Design review of the part built by this model. Coordinates are the model's own, in mm. Give positions to 0.01 mm unless a question says otherwise; leave off trailing zeros. Write each loop counter-clockwise with the first axis right and the second up, starting at its lowest first coordinate (ties: lowest second). Pieces come first, ordered by that corner, then holes. Notation, with made-up numbers: (-25.75, -27) -> (-8.75, -27) arc R32 cw to (-8.75, 10) -> close; hole circle Ø2 at (-17.75, 45). An arc over 180 degrees is marked (long way). Answer as a JSON object with one key per item and string values.
```python
from build123d import *

# Parameters (mm, degrees)
BOSS_EXTRUDE1_DEPTH     = 5
BOSS_EXTRUDE2_START     = 250
BOSS_EXTRUDE2_DEPTH     = 5
BOSS_EXTRUDE3_DEPTH     = 5
BOSS_EXTRUDE4_DEPTH     = 5
BOSS_EXTRUDE5_START     = -2.5
SKETCH12_R              = 5
BOSS_EXTRUDE5_DEPTH     = 2.5
BOSS_EXTRUDE6_START     = -20
SKETCH12_2_R            = 5
BOSS_EXTRUDE6_DEPTH     = 2.5
MIRROR2_START           = 250
MIRROR2_COPY_1_DEPTH    = 5
MIRROR2_COPY_2_DEPTH    = 5
MIRROR2_COPY_3_DEPTH    = 5
MIRROR2_START_2         = -2.5
MIRROR2_COPY_4_SKETCH_R = 5
MIRROR2_COPY_4_DEPTH    = 2.5
MIRROR2_START_3         = -20
MIRROR2_COPY_5_SKETCH_R = 5
MIRROR2_COPY_5_DEPTH    = 2.5
SKETCH13_W              = 25
SKETCH13_H              = 10
CUT_EXTRUDE1_DEPTH      = 5
FILLET1_R               = 2.5
SKETCH15_W              = 25
SKETCH15_H              = 10
CUT_EXTRUDE2_DEPTH      = 5
FILLET2_R               = 2.5


with BuildPart() as part:
    # Sketch2 → Boss-Extrude1 (new body, symmetric)
    with BuildSketch(Plane(origin=(0, 0, 0), x_dir=(1, 0, 0), z_dir=(0, 1, 0))):
        with BuildLine():
            Line((-272.5, 125), (-187.5, 125))
            ThreePointArc((-187.5, 125), (-62.5, 0), (-187.5, -125))
            Line((-187.5, -125), (-272.5, -125))
            ThreePointArc((-272.5, -125), (-300.784271247, -136.715728753), (-312.5, -165))
            Line((-312.5, -165), (-312.5, -175))
            Line((-312.5, -175), (312.5, -175))
            Line((312.5, -175), (312.5, -165))
            ThreePointArc((312.5, -165), (300.784271247, -136.715728753), (272.5, -125))
            Line((272.5, -125), (187.5, -125))
            ThreePointArc((187.5, -125), (62.5, 0), (187.5, 125))
            Line((187.5, 125), (272.5, 125))
            ThreePointArc((272.5, 125), (300.784271247, 136.715728753), (312.5, 165))
            Line((312.5, 165), (312.5, 175))
            Line((312.5, 175), (-312.5, 175))
            Line((-312.5, 175), (-312.5, 165))
            ThreePointArc((-312.5, 165), (-300.784271247, 136.715728753), (-272.5, 125))
        make_face()
    extrude(amount=BOSS_EXTRUDE1_DEPTH, both=True)

    # Sketch5 → Boss-Extrude2 (add)
    with BuildSketch(Plane(origin=(0, 0, 0), x_dir=(0, 0, -1), z_dir=(1, 0, 0)).offset(BOSS_EXTRUDE2_START)):
        with BuildLine():
            Line((175, 5), (125, 5))
            ThreePointArc((125, 5), (143.63387523, 48.296145769), (150, 95))
            Line((150, 95), (175, 95))
            Line((175, 95), (175, 5))
        make_face()
    boss_extrude2 = extrude(amount=BOSS_EXTRUDE2_DEPTH)

    # Sketch7 → Boss-Extrude3 (add)
    with BuildSketch(Plane(origin=(0, 95, 0), x_dir=(1, 0, 0), z_dir=(0, 1, 0))):
        with BuildLine():
            Line((260, 147.5), (137.5, 147.5))
            ThreePointArc((137.5, 147.5), (135.732233047, 148.232233047), (135, 150))
            Line((135, 150), (135, 155.899029492))
            ThreePointArc((135, 155.899029492), (135.394692651, 157.247243483), (136.454144772, 158.16975335))
            Line((136.454144772, 158.16975335), (172.44973726, 174.748686302))
            ThreePointArc((172.44973726, 174.748686302), (178.575849825, 176.804100302), (185, 177.5))
            Line((185, 177.5), (260, 177.5))
            Line((260, 177.5), (260, 147.5))
        make_face()
    boss_extrude3 = extrude(amount=-BOSS_EXTRUDE3_DEPTH)

    # Sketch10 → Boss-Extrude4 (add)
    with BuildSketch(Plane.ZY.offset(-150)):
        with BuildLine():
            Line((-175, 5), (-125, 5))
            ThreePointArc((-125, 5), (-141.779773176, 46.036236512), (-147.5, 90))
            Line((-147.5, 90), (-164.408734572, 90))
            ThreePointArc((-164.408734572, 90), (-167.06674937, 47.171344571), (-175, 5))
        make_face()
    boss_extrude4 = extrude(amount=-BOSS_EXTRUDE4_DEPTH)

    # Sketch12 → Boss-Extrude5 (add)
    with BuildSketch(Plane.XY.offset(-147.5).offset(BOSS_EXTRUDE5_START)):
        with BuildLine():
            Line((175, 95), (200, 95))
            Line((200, 95), (197.12585943, 105.209765716))
            ThreePointArc((197.12585943, 105.209765716), (187.5, 112.5), (177.87414057, 105.209765716))
            Line((177.87414057, 105.209765716), (175, 95))
        make_face()
        with Locations((187.5, 102.5)):
            Circle(SKETCH12_R, mode=Mode.SUBTRACT)
    boss_extrude5 = extrude(amount=-BOSS_EXTRUDE5_DEPTH)

    # Sketch12<2> → Boss-Extrude6 (add)
    with BuildSketch(Plane.XY.offset(-147.5).offset(BOSS_EXTRUDE6_START)):
        with BuildLine():
            Line((175, 95), (200, 95))
            Line((200, 95), (197.12585943, 105.209765716))
            ThreePointArc((197.12585943, 105.209765716), (187.5, 112.5), (177.87414057, 105.209765716))
            Line((177.87414057, 105.209765716), (175, 95))
        make_face()
        with Locations((187.5, 102.5)):
            Circle(SKETCH12_2_R, mode=Mode.SUBTRACT)
    boss_extrude6 = extrude(amount=-BOSS_EXTRUDE6_DEPTH)

    # Mirror1: Boss-Extrude2, Boss-Extrude3, Boss-Extrude4, Boss-Extrude5, Boss-Extrude6 across plane
    add(boss_extrude2.mirror(Plane.XY))
    add(boss_extrude3.mirror(Plane.XY))
    add(boss_extrude4.mirror(Plane.XY))
    add(boss_extrude5.mirror(Plane.XY))
    add(boss_extrude6.mirror(Plane.XY))

    # Mirror2: Boss-Extrude2, Boss-Extrude3, Boss-Extrude4, Boss-Extrude5, Boss-Extrude6 across plane
    add(boss_extrude2.mirror(Plane(origin=(0, 0, 0), x_dir=(0, 0, 1), z_dir=(1, 0, 0))))
    add(boss_extrude3.mirror(Plane(origin=(0, 0, 0), x_dir=(0, 0, 1), z_dir=(1, 0, 0))))
    add(boss_extrude4.mirror(Plane(origin=(0, 0, 0), x_dir=(0, 0, 1), z_dir=(1, 0, 0))))
    add(boss_extrude5.mirror(Plane(origin=(0, 0, 0), x_dir=(0, 0, 1), z_dir=(1, 0, 0))))
    add(boss_extrude6.mirror(Plane(origin=(0, 0, 0), x_dir=(0, 0, 1), z_dir=(1, 0, 0))))

    # Mirror2 copy 1 sketch → Mirror2 copy 1 (add)
    with BuildSketch(Plane.ZY.offset(MIRROR2_START)):
        with BuildLine():
            Line((175, 5), (125, 5))
            ThreePointArc((125, 5), (143.63387523, 48.296145769), (150, 95))
            Line((150, 95), (175, 95))
            Line((175, 95), (175, 5))
        make_face()
    extrude(amount=MIRROR2_COPY_1_DEPTH)

    # Mirror2 copy 2 sketch → Mirror2 copy 2 (add)
    with BuildSketch(Plane(origin=(0, 95, 0), x_dir=(-1, 0, 0), z_dir=(0, 1, 0))):
        with BuildLine():
            Line((260, 147.5), (137.5, 147.5))
            ThreePointArc((137.5, 147.5), (135.732233047, 148.232233047), (135, 150))
            Line((135, 150), (135, 155.899029492))
            ThreePointArc((135, 155.899029492), (135.394692651, 157.247243483), (136.454144772, 158.16975335))
            Line((136.454144772, 158.16975335), (172.44973726, 174.748686302))
            ThreePointArc((172.44973726, 174.748686302), (178.575849825, 176.804100302), (185, 177.5))
            Line((185, 177.5), (260, 177.5))
            Line((260, 177.5), (260, 147.5))
        make_face()
    extrude(amount=-MIRROR2_COPY_2_DEPTH)

    # Mirror2 copy 3 sketch → Mirror2 copy 3 (add)
    with BuildSketch(Plane(origin=(-150, 0, 0), x_dir=(0, 0, -1), z_dir=(1, 0, 0))):
        with BuildLine():
            Line((-175, 5), (-125, 5))
            ThreePointArc((-125, 5), (-141.779773176, 46.036236512), (-147.5, 90))
            Line((-147.5, 90), (-164.408734572, 90))
            ThreePointArc((-164.408734572, 90), (-167.06674937, 47.171344571), (-175, 5))
        make_face()
    extrude(amount=-MIRROR2_COPY_3_DEPTH)

    # Mirror2 copy 4 sketch → Mirror2 copy 4 (add)
    with BuildSketch(Plane(origin=(0, 0, 147.5), x_dir=(-1, 0, 0), z_dir=(0, 0, -1)).offset(MIRROR2_START_2)):
        with BuildLine():
            Line((175, 95), (200, 95))
            Line((200, 95), (197.12585943, 105.209765716))
            ThreePointArc((197.12585943, 105.209765716), (187.5, 112.5), (177.87414057, 105.209765716))
            Line((177.87414057, 105.209765716), (175, 95))
        make_face()
        with Locations((187.5, 102.5)):
            Circle(MIRROR2_COPY_4_SKETCH_R, mode=Mode.SUBTRACT)
    extrude(amount=-MIRROR2_COPY_4_DEPTH)

    # Mirror2 copy 5 sketch → Mirror2 copy 5 (add)
    with BuildSketch(Plane(origin=(0, 0, 147.5), x_dir=(-1, 0, 0), z_dir=(0, 0, -1)).offset(MIRROR2_START_3)):
        with BuildLine():
            Line((175, 95), (200, 95))
            Line((200, 95), (197.12585943, 105.209765716))
            ThreePointArc((197.12585943, 105.209765716), (187.5, 112.5), (177.87414057, 105.209765716))
            Line((177.87414057, 105.209765716), (175, 95))
        make_face()
        with Locations((187.5, 102.5)):
            Circle(MIRROR2_COPY_5_SKETCH_R, mode=Mode.SUBTRACT)
    extrude(amount=-MIRROR2_COPY_5_DEPTH)

    # Sketch13 → Cut-Extrude1 (cut)
    with BuildSketch(Plane(origin=(0, 95, 0), x_dir=(1, 0, 0), z_dir=(0, 1, 0))):
        with Locations((187.5, -160)):
            Rectangle(SKETCH13_W, SKETCH13_H)
    extrude(amount=-CUT_EXTRUDE1_DEPTH, mode=Mode.SUBTRACT)

    # Fillet1
    fillet1_edges = [part.edges().sort_by_distance(p)[0] for p in [
        (200, 92.5, 155),
        (200, 92.5, 165),
        (175, 92.5, 165),
        (175, 92.5, 155),
    ]]
    fillet(fillet1_edges, radius=FILLET1_R)

    # Sketch15 → Cut-Extrude2 (cut)
    with BuildSketch(Plane(origin=(0, 95, 0), x_dir=(1, 0, 0), z_dir=(0, 1, 0))):
        with Locations((-187.5, 160)):
            Rectangle(SKETCH15_W, SKETCH15_H)
    extrude(amount=-CUT_EXTRUDE2_DEPTH, mode=Mode.SUBTRACT)

    # Fillet2
    fillet2_edges = [part.edges().sort_by_distance(p)[0] for p in [
        (-200, 92.5, -155),
        (-200, 92.5, -165),
        (-175, 92.5, -165),
        (-175, 92.5, -155),
    ]]
    fillet(fillet2_edges, radius=FILLET2_R)


solid = part.part
```
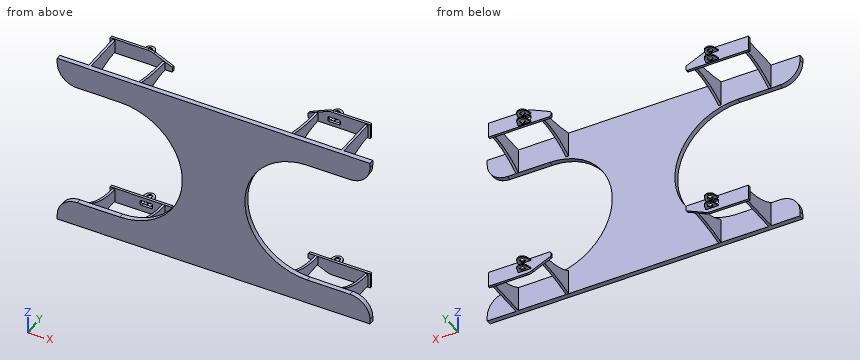
(1) We need section D-D, the plane z = 0. State the section outline as (x, y) points, then the cut area to 3 significant figures.
Here are the results:
{"outline": "(-62.5, -5) -> (62.5, -5) -> (62.5, 5) -> (-62.5, 5) -> close", "area": "1,250 mm²"}
(2) Clearance check with flat-ended pins moving along their axes: pin 1 (9 mm diameter, centred on x = 184.5, y = 107.5, fed in from -Z); pin 2 (5 mm diameter, centred on x = -238.5, y = -0.5, fed in from +Z); pin 3 (5.5 mm diameter, centred on y = 93.5, z = -153.5, fed in from -X). State where each tip first meets the part, or that it passes through.
Here are the results:
{"pin 1": "stops at z = -170", "pin 2": "stops at z = 175", "pin 3": "stops at x = -260"}
(3) We need section B-B, the plane y = 39. Give the number of separate pieces and of enclosed holes in the cut face, then the cut area to 3 significant figures.
Here are the results:
{"separate pieces": "8", "enclosed holes": "0", "area": "1,250 mm²"}
(4) We need section A-A, the plane x = 240. State the section outline as (y, z) points, then the cut area to 3 significant figures.
Here are the results:
{"outline": "(-5, -175) -> (5, -175) -> (5, -125) -> (-5, -125) -> close; (-5, 125) -> (5, 125) -> (5, 175) -> (-5, 175) -> close; (90, -177.5) -> (95, -177.5) -> (95, -147.5) -> (90, -147.5) -> close; (90, 147.5) -> (95, 147.5) -> (95, 177.5) -> (90, 177.5) -> close", "area": "1,300 mm²"}
(5) For line 1 along X through (y, z) = (12.5, -140); line 2 along Y through (x, z) = (187.5, 169.3); line 3 along Z through (x, y) = (-206, 1.5), list the stretches that pass through material, from the lowest coordinate up.
Here are the results:
{"line 1": "x = -255 to -250, -155 to -150, 150 to 155, 250 to 255", "line 2": "y = -5 to 5, 90 to 97.5, 107.5 to 112.5", "line 3": "z = -175 to -125, 125 to 175"}
